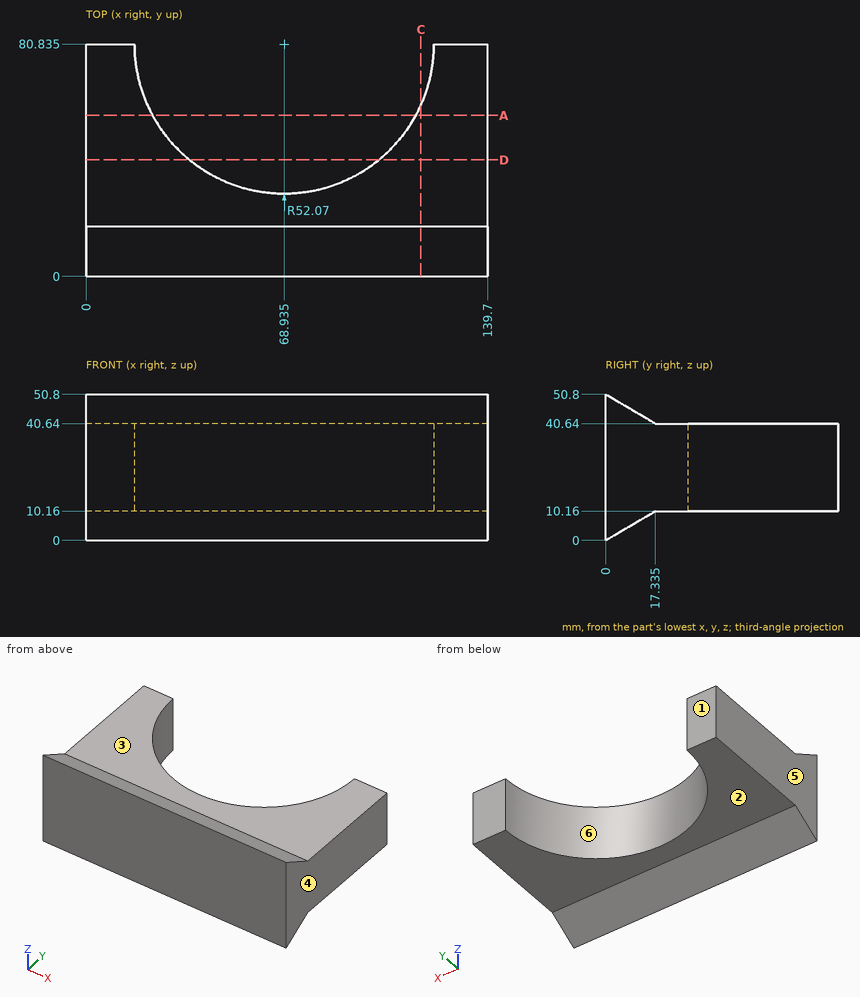
Answer from the drawing. Dimensions are ordinates in mm from the lowest x, y and z of the part. A direction names the side the tool comes from. Round coordinates to 2 decimals unless told otherwise and drop trailing zeros. Write each loop counter-clockwise with the first axis right and the second up, starting at its lowest first coordinate (ties: lowest second). Pieces come first, ordered by that corner, then holes.
1. The part is cut by section C-C, the plane x = 116.5. Determine the outline of the cut face in (y, z) (1 decimal), then the cut area to 3 significant figures.
2. The part is cut by section D-D, the plane y = 40.5. Determine the outline of the cut face in (x, z) (1 decimal), then the cut area to 3 significant figures.
3. Given pin 1 Ø1 at (y, z) = (68.5, 43) entering from -X; pin 2 Ø2 at (x, y) = (29.5, 22.5) entering from +Z, each flat-ended and moving along its own axis, determine where each tip first touches the part or whether it passes through.
4. Which of the six approach directions +Z, -Z, +X, -X, +Y, -Y give full straight-line access (tool end or side, diameter ignored) to the marked faces 1 and 2?
5. Determine the mould class of the marked faces 3, 4, 5 and 6 for opening direction X: pulls with the +X half, pulls with the -X half, needs draft (parallel to the pull), parting line crosses it, or undercut.
6. Straight lines are drawn through the part: L1, parallel to X at y = 78, z = 39; L2, parallel to Z at x = 125, y = 30; L3, parallel to X at y = 70, z = 10.5 (1 decimal). For each, find the intervals that lie inside material, in ascending order.
7. The part is cut by section A-A, the plane y = 56. Determine the outline of the cut face in (x, z), then the cut area to 3 significant figures.
Values:
1. outline: (0, 0) - (17.3, 10.2) - (59.6, 10.2) - (59.6, 40.6) - (17.3, 40.6) - (0, 50.8) - close
1. area: 1,990 mm2
2. outline: (0, 10.2) - (36, 10.2) - (36, 40.6) - (0, 40.6) - close; (101.9, 10.2) - (139.7, 10.2) - (139.7, 40.6) - (101.9, 40.6) - close
2. area: 2,250 mm2
3. pin 1: passes through
3. pin 2: stops at z = 40.64
4. face 1: +Z, -Z, +X, -X, +Y
4. face 2: -Z, +X, -X, +Y
5. face 3: needs draft
5. face 4: pulls with the +X half
5. face 5: pulls with the -X half
5. face 6: undercut
6. L1: x = 0 to 16.94, 120.93 to 139.7
6. L2: z = 10.16 to 40.64
6. L3: x = 0 to 18, 119.9 to 139.7
7. outline: (0, 10.16) - (23.17, 10.16) - (23.17, 40.64) - (0, 40.64) - close; (114.7, 10.16) - (139.7, 10.16) - (139.7, 40.64) - (114.7, 40.64) - close
7. area: 1,470 mm2
